Solid Edge part; units mm, degrees
sketch "Sketch1" plane through (0, 0, 0) normal (1, 0, 0) x (0, 1, 0)
  line L0 (74, 81.0476) -> (74, 0)
  line L1 (44, 80) -> (74, 81.0476)
  line L2 (44, 80) -> (44, 44.0365)
  line L3 (0, 42.5) -> (44, 44.0365)
  line L4 (0, 42.5) -> (0, 0)
  dimension "D1" = 44
  dimension "D2" = 74
revolve "RevolvedProtrusion1" add sketch "Sketch1" angle 360 about axis through (0, 0, 0) along (0, 1, 0)
sketch "Sketch2" plane through (0, 0, 0) normal (0, -1, 0) x (1, 0, 0)
  circle A0 centre (0, 0) radius 28
extrude "Cutout1" cut sketch "Sketch2" against normal blind 250.3843
fillet "Raccordi_grezzo" radius 6 4 edges at (0, 74, 81.0476) (0, 44, 80) (0, 44, 44.0365) (0, 0, 42.5)
properties material "Acciaio"
Read the model definition and answer for the solid it produces. Units are mm, in the model's axes. A direction names the side the tool comes from. Coordinates: 2 decimals unless noted, no trailing zeros. Write each loop counter-clockwise with the first axis right and the second up, starting at its lowest first coordinate (ties: lowest second). Pieces come first, ordered by that corner, then holes. Notation, with made-up numbers: M 9,-3.5 L 36,-3.5 A33 ccw 36,29.5 Z; hole C 3.5,-5.75 d6. An arc over 180 degrees is marked long. Use a Markdown table: item, result.
Q1. The part is cut by section A-A, the plane x = 0. Write down the section's boundary in (y, z), then the cut area to 3 significant figures.
Answer block:
| item | result |
|---|---|
| outline | M 0,-36.71 A6 ccw 5.79,-42.7 L 38.21,-43.83 A6 cw 44,-49.83 L 44,-74.21 A6 ccw 49.79,-80.2 L 67.79,-80.83 A6 ccw 74,-74.83 L 74,-28 L 0,-28 Z; M 0,28 L 74,28 L 74,74.83 A6 ccw 67.79,80.83 L 49.79,80.2 A6 ccw 44,74.21 L 44,49.83 A6 cw 38.21,43.83 L 5.79,42.7 A6 ccw 0,36.71 Z |
| area | 4,460 mm2 |
Q2. The part is cut by section D-D, the plane y = 12. Write down the section's boundary in (x, z), then the cut area to 3 significant figures.
Answer block:
| item | result |
|---|---|
| outline | C 0,0 d85.84; hole C 0,0 d56 |
| area | 3,320 mm2 |
Q3. The part is cut by section B-B, the plane z = 0. Write down the section's boundary in (x, y).
Answer block:
| item | result |
|---|---|
| outline | M -80.83,67.79 L -80.2,49.79 A6 ccw -74.21,44 L -49.83,44 A6 cw -43.83,38.21 L -42.7,5.79 A6 ccw -36.71,0 L -28,0 L -28,74 L -74.83,74 A6 ccw Z; M 28,0 L 36.71,0 A6 ccw 42.7,5.79 L 43.83,38.21 A6 cw 49.83,44 L 74.21,44 A6 ccw 80.2,49.79 L 80.83,67.79 A6 ccw 74.83,74 L 28,74 Z |
Q4. Straight lines are drawn through the part: L1, parallel to Y at x = 18.5, z = 50; L2, parallel to Z at x = 0, y = 35; L3, parallel to Z at x = 0, y = 36. For each, find the intervals that lie inside material, in ascending order. Write a range as [from, to].
Answer block:
| item | result |
|---|---|
| L1 | y = [44, 74] |
| L2 | z = [-43.72, -28], [28, 43.72] |
| L3 | z = [-43.76, -28], [28, 43.76] |
Q5. Each of these flat-tipped pins is pushed along its axis until it touches: pin 1 Ø6 at (x, z) = (58, -57) entering from +Y; pin 2 Ø2 at (y, z) = (33.5, 27.5) entering from -X; pin 3 Ø4 at (x, y) = (-16, 52.5) entering from +Z. Where does it stop, or does it pass through?
Answer block:
| item | result |
|---|---|
| pin 1 | stops at y = 72.88 |
| pin 2 | stops at x = -34.71 |
| pin 3 | stops at z = 79.07 |
Q6. Which of the six approach directions +Z, -Z, +X, -X, +Y, -Y give full straight-line access (tool end or side, diameter ignored) to faces 1 (the face through (-15, 44, 48)), 2 (the face through (1, 74, 32))?
Answer block:
| item | result |
|---|---|
| face 1 | -Y |
| face 2 | +Z, -Z, +X, -X, +Y |
Q7. The part is cut by section C-C, the plane y = 28. Write down the section's boundary in (x, z), then the cut area to 3 significant figures.
Answer block:
| item | result |
|---|---|
| outline | C 0,0 d86.96; hole C 0,0 d56 |
| area | 3,480 mm2 |
Q8. Determine the mould class of faces 3 (the face through (25.865, 36.482, -10.724)), 4 (the face through (-42.247, 22.227, -9.381)), 5 (the face through (-27, 0, -8)) for opening direction X: released by +X, released by -X, zero draft, split by the parting line, or undercut.
Answer block:
| item | result |
|---|---|
| face 3 | undercut |
| face 4 | split by the parting line |
| face 5 | zero draft |
